```python
from build123d import *

# Parameters (mm, degrees)
CROQUIS3_R                   = 25
SALIENTE_EXTRUIR1_DEPTH      = 463.3
CROQUIS5_R                   = 100
SALIENTE_EXTRUIR2_DEPTH      = 15
SALIENTE_EXTRUIR3_REACH      = 1699.123
SALIENTE_EXTRUIR3_END_RADIUS = 25
CROQUIS6_R                   = 25


with BuildPart() as part:
    # Croquis3 → Saliente-Extruir1 (new body)
    with BuildSketch(Plane(origin=(-202.746163562, 0, 0), x_dir=(0, 0, -1), z_dir=(1, 0, 0))):
        with Locations((-5751.601025747, 1500.190716107)):
            Circle(CROQUIS3_R)
    extrude(amount=-SALIENTE_EXTRUIR1_DEPTH)



with BuildPart() as body_2:
    # Croquis5 → Saliente-Extruir2 (new body)
    with BuildSketch(Plane(origin=(0, 775.966680828, 6979.147433935), x_dir=(1, 0, 0), z_dir=(0, -0.11050268429861657, -0.9938758256255157))):
        with Locations(Location((-469.396163562, -855.435934207, 0), (0, 0, 90))):
            Circle(CROQUIS5_R)
    extrude(amount=SALIENTE_EXTRUIR2_DEPTH)


with BuildPart() as part_1:
    add(part.part)

    add(body_2.part)  # Saliente-Extruir3 merges body 2
    # Saliente-Extruir3: up to this cylinder (the profile starts outside it)
    saliente_extruir3_end = Plane(origin=(-469.396164, 1500.190716107, 5751.601025747), z_dir=(1, 0, 0)) * Cylinder(SALIENTE_EXTRUIR3_END_RADIUS, 3449.246, mode=Mode.PRIVATE)
    # Croquis6 → Saliente-Extruir3 (add, up to the surface)
    with BuildSketch(Plane(origin=(0, 774.309140563, 6964.239296551), x_dir=(1, 0, 0), z_dir=(0, -0.11050268429861657, -0.9938758256255156)), mode=Mode.PRIVATE) as saliente_extruir3_sk1:
        with Locations(Location((-469.396163562, -855.435934207, 0), (0, 0, 270))):
            Circle(CROQUIS6_R)
    saliente_extruir3_tool1 = extrude(saliente_extruir3_sk1.sketch, amount=SALIENTE_EXTRUIR3_REACH, mode=Mode.PRIVATE) - saliente_extruir3_end
    add(saliente_extruir3_tool1.solids().sort_by_distance((-469.396164, 1624.506236, 6869.71133))[0])


solid = part_1.part
```
Build history of the part. All positions in model axes, mm. A direction names the side the tool comes from. Coordinates: 2 decimals unless noted, no trailing zeros. Order: outer loops, then holes, each group sorted by start corner. A loop starts at its lowest first (then second) coordinate and runs counter-clockwise, first axis right, second up. Notation, with made-up numbers: (-1.5, -39) -> (36.5, -39) arc R7 ccw to (36.5, -30) -> close; hole circle Ø8 at (85, 0.5). An arc over 180 degrees is marked (long way). Answer in a Markdown table with one row per item. Add a question column.
Q1. Band-saw the part on A-A, the plane x = -546.5. List the corners of the cut face in (y, z).
Q2. Band-saw the part on B-B, the plane x = -432. List the corners of the cut face in (y, z), then the cut area to 3 significant figures.
Q3. Which spindle directions (+Z, -Z, +X, -X, +Y, -Y) get a long thin tool onto all of the face, cutting with end or side? Do faces 5 (the face through (-431.153, 1507.7, 5727.755)), 6 (the face through (-666.046, 1501, 5752)). Say none if no direction does.
Q4. Band-saw the part on C-C, the plane x = -596. List the corners of the cut face in (y, z), then the cut area to 3 significant figures.
Q5. Wall check: line 1 along Z through (x, y) = (-593.5, 1503.5); line 2 along Z through (x, y) = (-279.5, 1498); line 3 along X through (y, z) = (1521.5, 6062). Give the ranges that are in metal, low to high. Write a range as [from, to].
Q6. Mould opens along Z. For faces 1 (the face through (-202.746, 1501, 5752)), 2 (the face through (-470.796, 1627.555, 6884.465)), 3 (the face through (-473.79, 1724.64, 6866.23)), 4 (the face through (-448.32, 1576.58, 6317)) say: +Z half, -Z half, draft (parallel to the pull), parting line (faces both ways), or undercut.
Answers follow:
| question | item | result |
|---|---|---|
| 1 | outline | circle Ø50 at (1500.19, 5751.6); (1561.22, 6876.75) -> (1687.8, 6862.67) -> (1689.45, 6877.58) -> (1562.87, 6891.66) -> close |
| 2 | outline | circle Ø50 at (1500.19, 5751.6); (1532.33, 6879.96) -> (1716.68, 6859.46) -> (1718.34, 6874.37) -> (1533.99, 6894.87) -> close |
| 2 | area | 4,750 mm^2 |
| 3 | face 5 | none |
| 3 | face 6 | +Z, -Z, -X, +Y, -Y |
| 4 | outline | circle Ø50 at (1500.19, 5751.6) |
| 4 | area | 1,960 mm^2 |
| 5 | line 1 | [5726.82, 5776.38] |
| 5 | line 2 | [5726.7, 5776.5] |
| 5 | line 3 | [-490.68, -448.12] |
| 6 | face 1 | draft |
| 6 | face 2 | +Z half |
| 6 | face 3 | parting line |
| 6 | face 4 | undercut |
